Check sheet for the modelled part. Datum: model origin and axes. Units: mm. A direction names the side the tool comes from. Coordinates: 2 decimals unless noted, no trailing zeros. Loops run counter-clockwise (first coordinate to the right, second up) from the corner with the lowest first, then second, coordinate; pieces in that order, holes last. Notation, with made-up numbers: (75.25, 41) - (85.25, 41) arc R5 cw to (85.25, 50) - close; hole circle Ø11 at (-14.75, 50). An arc over 180 degrees is marked (long way). Write each question's results on one line, items separated by ' | '. Start each with the question number.
1. Draft check along Z on faces 4 (the face through (-33, 12, 23.35)), 5 (the face through (33.035, 0.705, 32.173)), 6 (the face through (0, 14, 17)), 7 (the face through (33.03, -4.46, 34.54)). Enter one of: released by +Z, released by -Z, zero draft, split by the parting line, or undercut.
2. Cross-section at A-A (z = 15.5). Record the cut outline in (x, y).
3. Cross-section at B-B (z = 20). Record the cut outline in (x, y) (3 decimals).
4. Cross-section at C-C (x = 20.4). Record the cut outline in (y, z).
5. Cross-section at D-D (y = -7.25). Record the cut outline in (x, z), and give its area (4 significant figures).
6. Gauge pin test, flat ends, axial feed: P1, Ø2, axis at x = 0, y = -11.5, coming from the +Z side; P2, Ø2, axis at y = -4.3, z = 33.3, coming from the -X side; P3, Ø5, axis at y = 0, z = 29, coming from the +X side; P4, Ø1.6, axis at x = 0, y = 0, coming from the +Z side. Record the tip position at first contact, or that the pin passes through.
7. Tool access check on faces 1 (the face through (16, -11, 23.35)), 2 (the face through (-35.5, 0, 17)), 3 (the face through (-33.035, -3.379, 25.545)). Record the directions out of +Z, -Z, +X, -X, +Y, -Y that give a thin tool (end or side, any length) a straight path to the whole face; none if there is none.
8. Thickness scan on line 1 (Z direction, x = -34, y = 4.3); line 2 (X direction, y = -11.5, z = 28.5); line 3 (Y direction, x = 0, z = 26). Record the ranges inside material, lowest first. Write a range as [from, to].
```python
from build123d import *

# Parameters (mm, degrees)
F0_W      = 71
F0_H      = 28
F0_R      = 5
F0_W_2    = 2
F0_H_2    = 1
F0_H_3    = 16
F1_DEPTH  = 5
F2_DEPTH  = 35.35
F3_DEPTH  = 17.5
F4_R      = 0.5
F5_DEPTH  = 5
F6_W      = 0.5
F6_H      = 18
F11_DEPTH = 12
F12_R     = 1
F9_R      = 1.25
F14_DEPTH = 5
F13_R     = 1.25
F15_DEPTH = 5


with BuildPart() as f1:
    # F0 (on Top) → F1 (new body)
    with BuildSketch(Plane.XY):
        Rectangle(F0_W, F0_H)
        Polygon((-1, -9), (-30.5, -9), (-30.5, 9), (-1, 9), (1, 9), (30.5, 9), (30.5, -9), (1, -9), align=None, mode=Mode.SUBTRACT)
        Polygon((-30.5, 9), (-30.5, -9), (-1, -9), (-1, -8), (-1, 8), (-1, 9), align=None)
        with Locations((-20.4, 0)):
            Circle(F0_R, mode=Mode.SUBTRACT)
        with Locations((-9, 0)):
            Circle(F0_R, mode=Mode.SUBTRACT)
        Polygon((1, -8), (1, -9), (30.5, -9), (30.5, 9), (1, 9), (1, 8), align=None)
        with Locations((9, 0)):
            Circle(F0_R, mode=Mode.SUBTRACT)
        with Locations((20.4, 0)):
            Circle(F0_R, mode=Mode.SUBTRACT)
        with Locations((-20.4, 0)):
            Circle(F0_R)
        with Locations((-9, 0)):
            Circle(F0_R)
        with Locations((9, 0)):
            Circle(F0_R)
        with Locations((20.4, 0)):
            Circle(F0_R)
        with Locations((0, 8.5)):
            Rectangle(F0_W_2, F0_H_2)
        with Locations((0, -8.5)):
            Rectangle(F0_W_2, F0_H_2)
        Rectangle(F0_W_2, F0_H_3)
    extrude(amount=F1_DEPTH)

    # F0 (on Top) → F2 (join)
    with BuildSketch(Plane.XY):
        Rectangle(F0_W, F0_H)
        Polygon((-1, -9), (-30.5, -9), (-30.5, 9), (-1, 9), (1, 9), (30.5, 9), (30.5, -9), (1, -9), align=None, mode=Mode.SUBTRACT)
        with Locations((0, 8.5)):
            Rectangle(F0_W_2, F0_H_2)
        with Locations((0, -8.5)):
            Rectangle(F0_W_2, F0_H_2)
    extrude(amount=F2_DEPTH)

    # F0 (on Top) → F3 (join)
    with BuildSketch(Plane.XY):
        Rectangle(F0_W_2, F0_H_3)
    extrude(amount=F3_DEPTH)

    # F4
    f4_edges = [f1.edges().sort_by_distance(p)[0] for p in [
        (-1, 9, 20.175),
        (1, 9, 20.175),
        (-1, -9, 20.175),
        (1, -9, 20.175),
    ]]
    fillet(f4_edges, radius=F4_R)

    # F0 (on Top) → F5 (cut)
    with BuildSketch(Plane.XY):
        with Locations((-20.4, 0)):
            Circle(F0_R)
        with Locations((20.4, 0)):
            Circle(F0_R)
        with Locations((-9, 0)):
            Circle(F0_R)
        with Locations((9, 0)):
            Circle(F0_R)
    extrude(amount=F5_DEPTH, mode=Mode.SUBTRACT)

    # F6 (on Front) → F7 (revolve)
    with BuildSketch(Plane.XZ):
        Polygon((-14, 30), (-14, 0), (-13, 0), (-13, 18), (-13, 23), (-13, 30), align=None)
        Polygon((-13, 23), (-13, 18), (-12.5, 18), (-12.175, 18), (-12.175, 23), align=None)
        with Locations((-12.75, 9)):
            Rectangle(F6_W, F6_H)
    revolve(axis=Axis((-9, 0, 20.5), (0, 0, -1)))

    # F6 (on Front) → F8 (revolve)
    with BuildSketch(Plane.XZ):
        Polygon((12.5, 18), (13, 18), (13, 23), (12.175, 23), (12.175, 18), align=None)
        Polygon((13, 23), (13, 18), (13, 0), (14, 0), (14, 30), (13, 30), align=None)
        with Locations((12.75, 9)):
            Rectangle(F6_W, F6_H)
    revolve(axis=Axis((9, 0, 20.5), (0, 0, -1)))

    # F10 (on face) → F11 (cut)
    with BuildSketch(Plane.XY.offset(35.35)):
        with BuildLine():
            ThreePointArc((-33, 10.25), (-32.1161165235, 10.6161165235), (-31.75, 11.5))
            Line((-31.75, 11.5), (-33, 11.5))
            Line((-33, 11.5), (-33, 10.25))
        make_face()
        with BuildLine():
            Line((-33, 11.5), (-31.75, 11.5))
            ThreePointArc((-31.75, 11.5), (-33.8838834765, 12.3838834765), (-33, 10.25))
            Line((-33, 10.25), (-33, 11.5))
        make_face()
        with BuildLine():
            ThreePointArc((-15.25, 11.5), (-16.5, 12.75), (-17.75, 11.5))
            Line((-17.75, 11.5), (-15.25, 11.5))
        make_face()
        with BuildLine():
            Line((-15.25, 11.5), (-17.75, 11.5))
            ThreePointArc((-17.75, 11.5), (-16.5, 10.25), (-15.25, 11.5))
        make_face()
        with BuildLine():
            ThreePointArc((1.25, 11.5), (0, 12.75), (-1.25, 11.5))
            Line((-1.25, 11.5), (1.25, 11.5))
        make_face()
        with BuildLine():
            Line((1.25, 11.5), (-1.25, 11.5))
            ThreePointArc((-1.25, 11.5), (0, 10.25), (1.25, 11.5))
        make_face()
        with BuildLine():
            ThreePointArc((17.75, 11.5), (16.5, 12.75), (15.25, 11.5))
            Line((15.25, 11.5), (17.75, 11.5))
        make_face()
        with BuildLine():
            Line((17.75, 11.5), (15.25, 11.5))
            ThreePointArc((15.25, 11.5), (16.5, 10.25), (17.75, 11.5))
        make_face()
        with BuildLine():
            Line((33, 11.5), (31.75, 11.5))
            ThreePointArc((31.75, 11.5), (32.1161165235, 10.6161165235), (33, 10.25))
            Line((33, 10.25), (33, 11.5))
        make_face()
        with BuildLine():
            ThreePointArc((34.25, 11.5), (33, 12.75), (31.75, 11.5))
            Line((31.75, 11.5), (33, 11.5))
            Line((33, 11.5), (33, 10.25))
            ThreePointArc((33, 10.25), (33.8838834765, 10.6161165235), (34.25, 11.5))
        make_face()
        with BuildLine():
            ThreePointArc((-31.75, -11.5), (-32.1161165235, -10.6161165235), (-33, -10.25))
            Line((-33, -10.25), (-33, -11.5))
            Line((-33, -11.5), (-31.75, -11.5))
        make_face()
        with BuildLine():
            Line((-33, -11.5), (-33, -10.25))
            ThreePointArc((-33, -10.25), (-33.8838834765, -12.3838834765), (-31.75, -11.5))
            Line((-31.75, -11.5), (-33, -11.5))
        make_face()
        with BuildLine():
            ThreePointArc((-15.25, -11.5), (-16.5, -10.25), (-17.75, -11.5))
            Line((-17.75, -11.5), (-15.25, -11.5))
        make_face()
        with BuildLine():
            Line((-15.25, -11.5), (-17.75, -11.5))
            ThreePointArc((-17.75, -11.5), (-16.5, -12.75), (-15.25, -11.5))
        make_face()
        with BuildLine():
            ThreePointArc((1.25, -11.5), (0, -10.25), (-1.25, -11.5))
            Line((-1.25, -11.5), (1.25, -11.5))
        make_face()
        with BuildLine():
            Line((1.25, -11.5), (-1.25, -11.5))
            ThreePointArc((-1.25, -11.5), (0, -12.75), (1.25, -11.5))
        make_face()
        with BuildLine():
            ThreePointArc((17.75, -11.5), (16.5, -10.25), (15.25, -11.5))
            Line((15.25, -11.5), (17.75, -11.5))
        make_face()
        with BuildLine():
            Line((17.75, -11.5), (15.25, -11.5))
            ThreePointArc((15.25, -11.5), (16.5, -12.75), (17.75, -11.5))
        make_face()
        with BuildLine():
            Line((33, -11.5), (33, -10.25))
            ThreePointArc((33, -10.25), (32.1161165235, -10.6161165235), (31.75, -11.5))
            Line((31.75, -11.5), (33, -11.5))
        make_face()
        with BuildLine():
            ThreePointArc((34.25, -11.5), (33.8838834765, -10.6161165235), (33, -10.25))
            Line((33, -10.25), (33, -11.5))
            Line((33, -11.5), (31.75, -11.5))
            ThreePointArc((31.75, -11.5), (33, -12.75), (34.25, -11.5))
        make_face()
    extrude(amount=-F11_DEPTH, mode=Mode.SUBTRACT)

    # F12
    f12_edges = [f1.edges().sort_by_distance(p)[0] for p in [
        (-30.5, -9, 20.175),
        (-30.5, 9, 20.175),
        (30.5, 9, 20.175),
        (30.5, -9, 20.175),
    ]]
    fillet(f12_edges, radius=F12_R)

    # F9 (on face) → F14 (cut)
    with BuildSketch(Plane(origin=(-35.5, 0, 0), x_dir=(0, -1, 0), z_dir=(-1, 0, 0))):
        with BuildLine():
            Line((0, 29), (3.25, 29))
            ThreePointArc((3.25, 29), (2.2980970389, 31.2980970389), (0, 32.25))
            Line((0, 32.25), (0, 29))
        make_face()
        with BuildLine():
            ThreePointArc((0, 25.75), (2.2980970389, 26.7019029611), (3.25, 29))
            Line((3.25, 29), (0, 29))
            Line((0, 29), (0, 25.75))
        make_face()
        with BuildLine():
            Line((0, 29), (0, 32.25))
            ThreePointArc((0, 32.25), (-2.2980970389, 31.2980970389), (-3.25, 29))
            Line((-3.25, 29), (0, 29))
        make_face()
        with BuildLine():
            ThreePointArc((-3.25, 29), (-2.2980970389, 26.7019029611), (0, 25.75))
            Line((0, 25.75), (0, 29))
            Line((0, 29), (-3.25, 29))
        make_face()
        with Locations((-4.3, 33.3)):
            Circle(F9_R)
        with Locations((-4.3, 24.7)):
            Circle(F9_R)
        with Locations((4.3, 33.3)):
            Circle(F9_R)
        with Locations((4.3, 24.7)):
            Circle(F9_R)
    extrude(amount=-F14_DEPTH, mode=Mode.SUBTRACT)

    # F13 (on face) → F15 (cut)
    with BuildSketch(Plane.YZ.offset(35.5)):
        with BuildLine():
            Line((-3.25, 29), (3.25, 29))
            ThreePointArc((3.25, 29), (0, 32.25), (-3.25, 29))
        make_face()
        with BuildLine():
            ThreePointArc((-3.25, 29), (0, 25.75), (3.25, 29))
            Line((3.25, 29), (-3.25, 29))
        make_face()
        with Locations((-4.3, 33.3)):
            Circle(F13_R)
        with Locations((-4.3, 24.7)):
            Circle(F13_R)
        with Locations((4.3, 33.3)):
            Circle(F13_R)
        with Locations((4.3, 24.7)):
            Circle(F13_R)
    extrude(amount=-F15_DEPTH, mode=Mode.SUBTRACT)


solid = f1.part
```
Established:
1) face 4: released by +Z | face 5: undercut | face 6: zero draft | face 7: undercut
2) outline: (-35.5, -14) - (35.5, -14) - (35.5, 14) - (-35.5, 14) - close; circle Ø10 at (-9, 0); circle Ø10 at (9, 0); hole (-30.5, -8) arc R1 ccw to (-29.5, -9) - (-1.5, -9) arc R0.5 ccw to (-1, -8.5) - (-1, 8.5) arc R0.5 ccw to (-1.5, 9) - (-29.5, 9) arc R1 ccw to (-30.5, 8) - close; hole circle Ø7 at (-9, 0); hole (1, -8.5) arc R0.5 ccw to (1.5, -9) - (29.5, -9) arc R1 ccw to (30.5, -8) - (30.5, 8) arc R1 ccw to (29.5, 9) - (1.5, 9) arc R0.5 ccw to (1, 8.5) - close; hole circle Ø7 at (9, 0)
3) outline: (-35.5, -14) - (35.5, -14) - (35.5, 14) - (-35.5, 14) - close; circle Ø10 at (-9, 0); circle Ø10 at (9, 0); hole (-30.5, -8) arc R1 ccw to (-29.5, -9) - (-1.5, -9) arc R0.5 ccw to (-1, -8.5) - (-1, -8) - (1, -8) - (1, -8.5) arc R0.5 ccw to (1.5, -9) - (29.5, -9) arc R1 ccw to (30.5, -8) - (30.5, 8) arc R1 ccw to (29.5, 9) - (1.5, 9) arc R0.5 ccw to (1, 8.5) - (1, 8) - (-1, 8) - (-1, 8.5) arc R0.5 ccw to (-1.5, 9) - (-29.5, 9) arc R1 ccw to (-30.5, 8) - close; hole circle Ø6.35 at (-9, 0); hole circle Ø6.35 at (9, 0)
4) outline: (-14, 0) - (-5, 0) - (-5, 5) - (-9, 5) - (-9, 35.35) - (-14, 35.35) - close; (5, 0) - (14, 0) - (14, 35.35) - (9, 35.35) - (9, 5) - (5, 5) - close
5) outline: (-35.5, 0) - (35.5, 0) - (35.5, 35.35) - (30.5, 35.35) - (30.5, 5) - (1, 5) - (1, 17.5) - (-1, 17.5) - (-1, 5) - (-30.5, 5) - (-30.5, 35.35) - (-35.5, 35.35) - close | area: 683.5 mm^2
6) P1: z = 23.35 | P2: through | P3: x = 14 | P4: z = 17.5
7) face 1: +Z | face 2: +Z, -Z, -X, +Y, -Y | face 3: -X
8) line 1: [0, 23.45], [25.95, 32.05], [34.55, 35.35] | line 2: [-35.5, -34.25], [-31.75, -17.75], [-15.25, -1.25], [1.25, 15.25], [17.75, 31.75], [34.25, 35.5] | line 3: [-14, -12.75], [-10.25, -8], [8, 10.25], [12.75, 14]
